```python
from build123d import *

# Parameters (mm, degrees)
ESQUISSE1_R                  = 85
BOSS_EXTRU_1_DEPTH           = 3
ESQUISSE2_R                  = 70
ENL_V_MAT_EXTRU_1_DEPTH      = 3
ESQUISSE3_R                  = 1.5
ENL_V_MAT_EXTRU_2_DEPTH      = 3
R_P_TITION_CIRCULAIRE1_COUNT = 6
CONG_1_R                     = 1


with BuildPart() as part:
    # Esquisse1 → Boss.-Extru.1 (new body)
    with BuildSketch(Plane(origin=(0, 0, 0), x_dir=(1, 0, 0), z_dir=(0, 1, 0))):
        with Locations(Location((0, 0, 0), (0, 0, 270))):
            Circle(ESQUISSE1_R)
    extrude(amount=BOSS_EXTRU_1_DEPTH)

    # Esquisse2 → Enlèv. mat.-Extru.1 (cut)
    with BuildSketch(Plane(origin=(0, 3, 0), x_dir=(1, 0, 0), z_dir=(0, 1, 0))):
        with Locations(Location((0, 0, 0), (0, 0, 270))):
            Circle(ESQUISSE2_R)
    extrude(amount=-ENL_V_MAT_EXTRU_1_DEPTH, mode=Mode.SUBTRACT)

    # Esquisse3 → Enlèv. mat.-Extru.2 (cut)
    with BuildSketch(Plane(origin=(0, 3, 0), x_dir=(1, 0, 0), z_dir=(0, 1, 0))):
        with Locations(Location((80, 0, 0), (0, 0, 270))):
            Circle(ESQUISSE3_R)
    enl_v_mat_extru_2 = extrude(amount=-ENL_V_MAT_EXTRU_2_DEPTH, mode=Mode.SUBTRACT)

    # Répétition circulaire1: Enlèv. mat.-Extru.2 ×6 about axis
    r_p_tition_circulaire1_axis = Axis((0, 0, 0), (0, 1, 0))
    for i in range(1, R_P_TITION_CIRCULAIRE1_COUNT):
        add(enl_v_mat_extru_2.rotate(r_p_tition_circulaire1_axis, i * 360 / R_P_TITION_CIRCULAIRE1_COUNT), mode=Mode.SUBTRACT)

    # Congé1
    cong_1_edges = [part.edges().sort_by_distance(p)[0] for p in [
        (0, 3, -85),
        (0, 3, -70),
    ]]
    fillet(cong_1_edges, radius=CONG_1_R)


solid = part.part
```
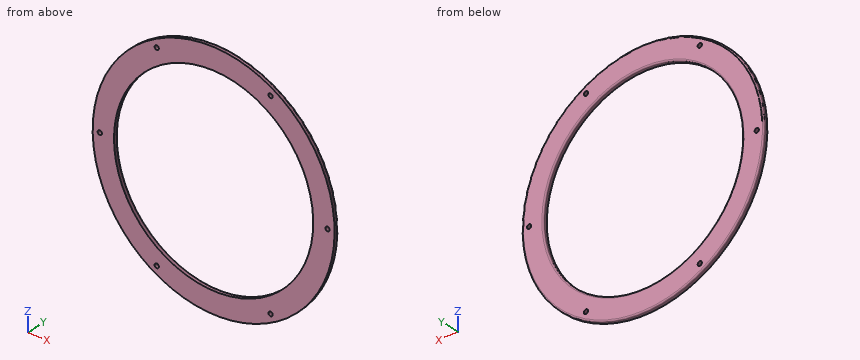
Model file for the job. Use its own axes, mm. Coordinates: 2 decimals unless noted, no trailing zeros. Order: outer loops, then holes, each group sorted by start corner. A loop starts at its lowest first (then second) coordinate and runs counter-clockwise, first axis right, second up. Notation, with made-up numbers: M -36,-11 L 13,-11 A20 cw 13,-2 Z; hole C 73.25,-35.75 d1. An arc over 180 degrees is marked long. Answer as CSV lines item,"result".
(1) Flat gauge pin, fed straight in: pin 1 (1 mm diameter, centred on y = 0.5, z = 44.5, fed in from +X). Where does the tip first touch, or does it go through?
Geometry says:
pin 1,"stops at x = 72.73"
(2) Band-saw the part on A-A, the plane y = 0.9. List the corners of the cut face in (x, z), then the cut area to 3 significant figures.
Geometry says:
outline,"C 0,0 d170; hole C -80,0 d3; hole C 0,0 d140; hole C -40,-69.28 d3; hole C -40,69.28 d3; hole C 40,-69.28 d3; hole C 40,69.28 d3; hole C 80,0 d3"
area,"7,260 mm2"
(3) Wall check: line 1 along X through (y, z) = (1.25, 0); line 2 along X through (y, z) = (2.45, -70.5); line 3 along X through (y, z) = (2.05, -60). Give the ranges that are in metal, low to high.
Geometry says:
line 1,"x = -85 to -81.5, -78.5 to -70, 70 to 78.5, 81.5 to 85"
line 2,"x = -47.29 to -40.88, -39.12 to 39.12, 40.88 to 47.29"
line 3,"x = -60.21 to -36.06, 36.06 to 60.21"
